CAD build for the part. Positions are in the model's coordinates, mm. Face numbers are marked on the shaded views. A direction names the side the tool comes from. Round coordinates to 2 decimals unless told otherwise and drop trailing zeros. Loops run counter-clockwise (first coordinate to the right, second up) from the corner with the lowest first, then second, coordinate; pieces in that order, holes last. Notation, with made-up numbers: M 54,-8.5 L 63,-8.5 A22 cw 63,12.5 Z; hole C -31.75,34.5 d7. An arc over 180 degrees is marked long. Use one line per item in the form item = value.
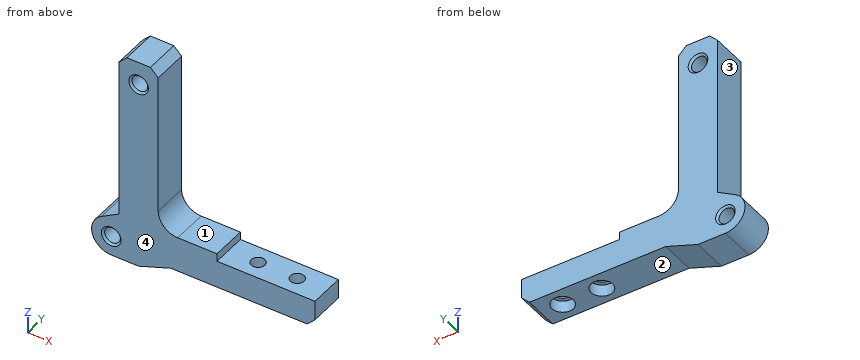
from build123d import *

# Parameters (mm, degrees)
F0_R           = 2
F1_DEPTH       = 4.5
F2_SIZE        = 0.5
F3_SIZE        = 2
F4_R           = 5
F6_D           = 3.5
F6_CBORE_D     = 5.5
F6_CBORE_DEPTH = 3


with BuildPart() as f1:
    # F0 (on Front) → F1 (new body, symmetric)
    with BuildSketch(Plane.XZ):
        with BuildLine():
            Line((2, 6.928203), (-2.5, 4.330127))
            ThreePointArc((-2.5, 4.330127), (-4.829629, -1.294095), (0, -5))
            Line((0, -5), (7, -5))
            Line((7, -5), (15.242432, -2))
            Line((15.242432, -2), (52, -2))
            Line((52, -2), (52, 5))
            Line((52, 5), (27, 5))
            Line((27, 5), (27, 7))
            Line((27, 7), (12, 7))
            Line((12, 7), (12, 50))
            Line((12, 50), (2, 50))
            Line((2, 50), (2, 6.928203))
        make_face()
        Circle(F0_R, mode=Mode.SUBTRACT)
        with Locations((7, 44)):
            Circle(F0_R, mode=Mode.SUBTRACT)
    extrude(amount=F1_DEPTH, both=True)

    # F2
    f2_edges = [f1.edges().sort_by_distance(p)[0] for p in [
        (5, -4.5, 44),
        (-2, -4.5, 0),
        (5, 4.5, 44),
        (-2, 4.5, 0),
    ]]
    chamfer(f2_edges, length=F2_SIZE)

    # F3
    f3_edges = [f1.edges().sort_by_distance(p)[0] for p in [
        (12, 0, 50),
        (2, 0, 50),
        (52, 0, -2),
    ]]
    chamfer(f3_edges, length=F3_SIZE)

    # F4
    f4_edges = [f1.edges().sort_by_distance(p)[0] for p in [
        (12, 0, 7),
    ]]
    fillet(f4_edges, radius=F4_R)

    # F6 (through all)
    with Locations(Plane(origin=(0, 0, -2), x_dir=(1, 0, 0), z_dir=(0, 0, -1))):
        with Locations((44.5, 0), (34.5, 0)):
            CounterBoreHole(F6_D / 2, F6_CBORE_D / 2, F6_CBORE_DEPTH)


solid = f1.part
1. Cut at B-B on z = 44. Write the cut outline in (x, y).
Completed:
outline = M 2,-4.5 L 4.5,-4.5 L 5,-4 L 5,4 L 4.5,4.5 L 2,4.5 Z; M 9,-4 L 9.5,-4.5 L 12,-4.5 L 12,4.5 L 9.5,4.5 L 9,4 Z
2. Drop flat-ended pins along their axis: P1, Ø1.5, axis at x = 25, y = 1, coming from the +Z side; P2, Ø4.5, axis at y = -1, z = 24.5, coming from the +X side; P3, Ø3, axis at y = 1, z = 24.5, coming from the -X side. Give the stop position or say it passes through.
Completed:
P1 = 7
P2 = 12
P3 = 2
3. Tool access for the marked faces 1, 2, 3 and 4: list every direction of +Z, -Z, +X, -X, +Y, -Y with a clear straight run to the whole face (end or side of a thin tool).
Completed:
face_1 = +Z, +X, +Y, -Y
face_2 = -Z, +X, +Y, -Y
face_3 = +Z, -X, +Y, -Y
face_4 = +Z, -Z, +X, -X, -Y
4. Cut at C-C on z = -1. State how many separate pieces and enclosed holes the cut face has, and give its area (3 significant figures).
Completed:
separate_pieces = 2
enclosed_holes = 2
area = 424 mm2
5. Cut at A-A on x = 34.5. Write the cut outline in (y, z), and give its area (3 significant figures).
Completed:
outline = M -4.5,-2 L -2.75,-2 L -2.75,1 L -1.75,1 L -1.75,5 L -4.5,5 Z; M 1.75,1 L 2.75,1 L 2.75,-2 L 4.5,-2 L 4.5,5 L 1.75,5 Z
area = 32.5 mm2
6. Probe line 1 along X through (y, z) = (-2.75, 25); line 2 along Z through (x, y) = (21, -1.25); line 3 along Z through (x, y) = (40.5, 3.25). List the from-to ranges inside material, lowest first. Write a range as from..to.
Completed:
line_1 = 2..12
line_2 = -2..7
line_3 = -2..5
7. Cut at D-D on z = 16.5. Write the cut outline in (x, y), and give its area (3 significant figures).
Completed:
outline = M 2,-4.5 L 12,-4.5 L 12,4.5 L 2,4.5 Z
area = 90.0 mm2
